Design review of the part built by this model. Coordinates are the model's own, in mm. Face numbers are marked on the shaded views. A direction names the side the tool comes from. Coordinates: 2 decimals unless noted, no trailing zeros. Loops run counter-clockwise (first coordinate to the right, second up) from the corner with the lowest first, then second, coordinate; pieces in that order, holes last. Notation, with made-up numbers: (6, 50.25) -> (22, 50.25) arc R30 ccw to (22, 83.25) -> close; hole circle Ø3 at (6, -37.5). An arc over 180 degrees is marked (long way). Use one line per item in the form item = value. Start each with the question number.
1. For pin 1 (15.5 mm diameter, centred on x = -30.44, z = 48.5, fed in from +Y); pin 2 (8.5 mm diameter, centred on x = -29.5, z = -16.5, fed in from -Y), all flat-tipped, find the tip position at first contact; note any pin that passes through.
2. Consider section C-C (x = -26.5). State the section outline as (y, z) points, then the cut area to 3 significant figures.
3. The part is to be moulded in two halves that separate along X. For the marked faces 3, 4, 5 and 6, say which applies: released by +X, released by -X, zero draft, split by the parting line, or undercut.
4. Machinability: for the marked faces 1 and 2, which of the approach directions +Z, -Z, +X, -X, +Y, -Y give a long, thin tool a straight path to every point of the face, cutting with its end or side? Answer none if there is none.
5. Consider section A-A (y = -79.5). State the section outline as (x, z) points.
6. Consider section B-B (z = 44). State the section outline as (x, y) points.
7. Wall thickness on line 1 (Z direction, x = -28, y = -51); line 2 (X direction, y = -78, z = 51.5); line 3 (X direction, y = -59, z = -23.5): over which ranges is each line inside the solid? List them lowest first. Write a range as from..to.
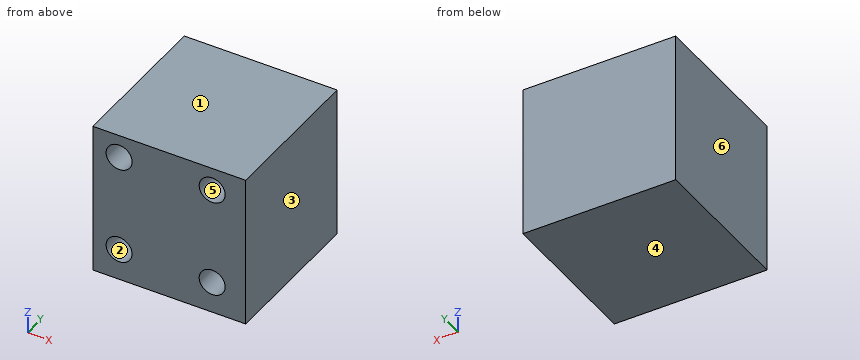
from build123d import *

# Parameters (mm, degrees)
F0_W     = 100
F0_H     = 100
F1_DEPTH = 100
F2_R     = 8.5
F3_DEPTH = 64
F5_ANGLE = 180


# Not quite as in the source:
# - a feature names something its author has since deleted; it is built from what else it names


with BuildPart() as f1:
    # F0 (on Front) → F1 (new body)
    with BuildSketch(Plane.XZ):
        with Locations((2.3967929184, 13.6052064598)):
            Rectangle(F0_W, F0_H)
    extrude(amount=F1_DEPTH)

    # F2 (on face) → F3 (cut)
    with BuildSketch(Plane.XZ.offset(100)):
        with Locations((30.443597585, 48.4984777868)):
            Circle(F2_R)
        with Locations((-30.443597585, -15.6539641321)):
            Circle(F2_R)
        with Locations((30.443597585, -15.6539641321)):
            Circle(F2_R)
        with Locations((-30.443597585, 48.4984777868)):
            Circle(F2_R)
    extrude(amount=-F3_DEPTH, mode=Mode.SUBTRACT)

    # F4 (on face) → F5 (revolve, cut)
    with BuildSketch(Plane.XZ.offset(100)):
        with BuildLine():
            Line((0, 0), (0, 26.83))
            ThreePointArc((0, 26.83), (-13.415, 13.415), (0, 0))
        make_face()
    revolve(axis=Axis((0, -100, 14.3139522988), (0, 0, 1)), revolution_arc=F5_ANGLE, mode=Mode.SUBTRACT)


solid = f1.part
Geometry check:
q1.pin_1 = 0
q1.pin_2 = -36
q2.outline = (-100, -36.39) -> (0, -36.39) -> (0, 63.61) -> (-100, 63.61) -> (-100, 56.03) -> (-36, 56.03) -> (-36, 40.97) -> (-100, 40.97) -> (-100, -8.12) -> (-36, -8.12) -> (-36, -23.18) -> (-100, -23.18) -> close
q2.area = 8,070 mm²
q3.face_3 = released by +X
q3.face_4 = zero draft
q3.face_5 = undercut
q3.face_6 = released by -X
q4.face_1 = +Z, +X, -X, +Y, -Y
q4.face_2 = -Y
q5.outline = (-47.6, -36.39) -> (52.4, -36.39) -> (52.4, 63.61) -> (-47.6, 63.61) -> close; hole circle Ø17 at (-30.44, -15.65); hole circle Ø17 at (-30.44, 48.5); hole circle Ø17 at (30.44, -15.65); hole circle Ø17 at (30.44, 48.5)
q6.outline = (-47.6, -100) -> (-37.66, -100) -> (-37.66, -36) -> (-23.23, -36) -> (-23.23, -100) -> (23.23, -100) -> (23.23, -36) -> (37.66, -36) -> (37.66, -100) -> (52.4, -100) -> (52.4, 0) -> (-47.6, 0) -> close
q7.line_1 = -36.39..-23.8, -7.51..40.36, 56.64..63.61
q7.line_2 = -47.6..-38.4, -22.49..22.49, 38.4..52.4
q7.line_3 = -47.6..-33.71, -27.17..27.17, 33.71..52.4
